Geometry check sheet. Reference: the model listing, model coordinates, mm. Face numbers are marked on the shaded views. A direction names the side the tool comes from. Coordinates: 2 decimals unless noted, no trailing zeros. Write each loop counter-clockwise with the first axis right and the second up, starting at its lowest first coordinate (ties: lowest second). Pieces come first, ordered by that corner, then holes. Notation, with made-up numbers: (74.5, 32) -> (116.5, 32) arc R24 ccw to (116.5, 61) -> close; hole circle Ø1 at (62.25, 14.25). An arc over 180 degrees is marked (long way). One line per question, with ' | ' between items.
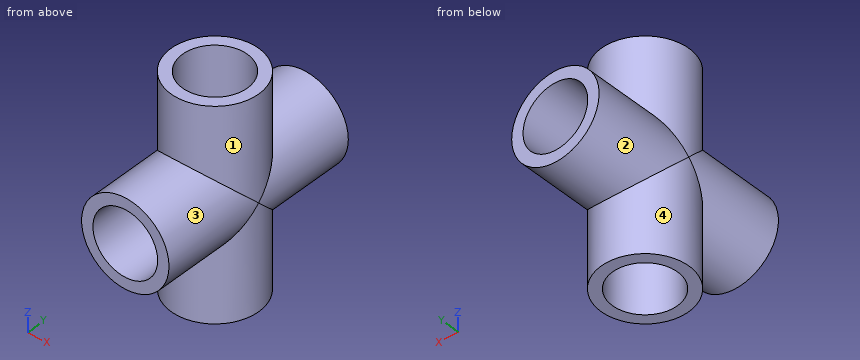
```python
from build123d import *

# Parameters (mm, degrees)
SKETCH1_R               = 10.668
SKETCH1_R_2             = 7.8994
BOSS_EXTRUDE1_DEPTH     = 50.8
SKETCH2_R               = 10.668
SKETCH2_R_2             = 7.8994
BOSS_EXTRUDE2_DEPTH     = 25.4
SKETCH3_R               = 7.8994
CUT_EXTRUDE1_DEPTH      = 51.8000001
SKETCH4_R               = 7.8994
CUT_EXTRUDE2_DEPTH      = 1.0000001
CUT_EXTRUDE2_DEPTH_BACK = 51.8000001


with BuildPart() as part:
    # Sketch1 → Boss-Extrude1 (new body)
    with BuildSketch(Plane.XY):
        Circle(SKETCH1_R)
        Circle(SKETCH1_R_2, mode=Mode.SUBTRACT)
    extrude(amount=BOSS_EXTRUDE1_DEPTH)

    # Sketch2 → Boss-Extrude2 (add, symmetric)
    with BuildSketch(Plane(origin=(0, 0, 0), x_dir=(1, 0, 0), z_dir=(0, 1, 0))):
        with Locations((0, -25.4)):
            Circle(SKETCH2_R)
        with Locations((0, -25.4)):
            Circle(SKETCH2_R_2, mode=Mode.SUBTRACT)
    extrude(amount=BOSS_EXTRUDE2_DEPTH, both=True)

    # Sketch3 → Cut-Extrude1 (cut, through all)
    with BuildSketch(Plane.XY.offset(50.8)):
        Circle(SKETCH3_R)
    extrude(amount=-CUT_EXTRUDE1_DEPTH, mode=Mode.SUBTRACT)

    # Sketch4 → Cut-Extrude2 (cut, two sides)
    with BuildSketch(Plane(origin=(0, 25.4, 0), x_dir=(1, 0, 0), z_dir=(0, 1, 0))) as cut_extrude2_sk:
        with Locations((0, -25.4)):
            Circle(SKETCH4_R)
    extrude(amount=CUT_EXTRUDE2_DEPTH, mode=Mode.SUBTRACT)
    extrude(cut_extrude2_sk.sketch, amount=-CUT_EXTRUDE2_DEPTH_BACK, mode=Mode.SUBTRACT)


solid = part.part
```
(1) Material ranges on line 1 (Z direction, x = 0, y = 11.75); line 2 (X direction, y = 0, z = 46), recorded low to high.
Answers below:
line 1: z = 14.73 to 17.5, 33.3 to 36.07 | line 2: x = -10.67 to -7.9, 7.9 to 10.67
(2) Cross-section at A-A (x = 0.75). Record the cut outline in (y, z).
Answers below:
outline: (-25.4, 14.76) -> (-10.64, 14.76) -> (-10.64, 0) -> (-7.86, 0) -> (-7.86, 17.54) -> (-25.4, 17.54) -> close; (-25.4, 33.26) -> (-7.86, 33.26) -> (-7.86, 50.8) -> (-10.64, 50.8) -> (-10.64, 36.04) -> (-25.4, 36.04) -> close; (7.86, 0) -> (10.64, 0) -> (10.64, 14.76) -> (25.4, 14.76) -> (25.4, 17.54) -> (7.86, 17.54) -> close; (7.86, 33.26) -> (25.4, 33.26) -> (25.4, 36.04) -> (10.64, 36.04) -> (10.64, 50.8) -> (7.86, 50.8) -> close
(3) Cross-section at C-C (y = 17). Record the cut outline in (x, z).
Answers below:
outline: circle Ø21.34 at (0, 25.4); hole circle Ø15.8 at (0, 25.4)
(4) Cross-section at B-B (z = 24.5). Record the cut outline in (x, y).
Answers below:
outline: (-10.63, -25.4) -> (-7.85, -25.4) -> (-7.85, -0.9) arc R7.9 cw to (-7.85, 0.9) -> (-7.85, 25.4) -> (-10.63, 25.4) -> (-10.63, 0.9) arc R10.67 ccw to (-10.63, -0.9) -> close; (7.85, -25.4) -> (10.63, -25.4) -> (10.63, -0.9) arc R10.67 ccw to (10.63, 0.9) -> (10.63, 25.4) -> (7.85, 25.4) -> (7.85, 0.9) arc R7.9 cw to (7.85, -0.9) -> close
(5) Depth check by flat-ended pin: P1, Ø1.5, axis at x = -3.5, y = -19, coming from the +Z side; P2, Ø1.5, axis at x = 4, y = 15, coming from the +Z side; P3, Ø9.5, axis at x = 0, y = 0, coming from the +Z side; P4, Ø4, axis at x = 7.5, y = 13, coming from the -Z side. Enter the tip coordinate at first touch or a pass-through.
Answers below:
P1: stops at z = 35.71 | P2: stops at z = 35.56 | P3: passes through | P4: stops at z = 16.26
(6) Cross-section at D-D (z = 16). Record the cut outline in (x, y).
Answers below:
outline: (-5.04, -25.4) -> (5.04, -25.4) -> (5.04, -9.4) arc R10.67 ccw to (5.04, 9.4) -> (5.04, 25.4) -> (-5.04, 25.4) -> (-5.04, 9.4) arc R10.67 ccw to (-5.04, -9.4) -> close; hole circle Ø15.8 at (0, 0)
(7) Tool access check on the marked faces 1, 2, 3 and 4. Record the directions out of +Z, -Z, +X, -X, +Y, -Y that give a thin tool (end or side, any length) a straight path to the whole face; none if there is none.
Answers below:
face 1: +Z | face 2: +Y | face 3: -Y | face 4: -Z
